from build123d import *

# Parameters (mm, degrees)
F0_W     = 50.8
F0_H     = 43.18
F1_DEPTH = 30.48
F2_R     = 16.51
F3_W     = 40.64
F3_H     = 20.32
F4_DEPTH = 38.1
F6_DEPTH = 2.54
F7_R     = 33.02
F8_R     = 9.525
F9_DEPTH = 25.4


with BuildPart() as f1:
    # F0 (on Front) → F1 (new body)
    with BuildSketch(Plane.XZ):
        with Locations((25.4, -21.59)):
            Rectangle(F0_W, F0_H)
    extrude(amount=F1_DEPTH)

    # F2
    f2_edges = [f1.edges().sort_by_distance(p)[0] for p in [
        (50.8, -15.24, -43.18),
    ]]
    fillet(f2_edges, radius=F2_R)

    # F3 (on face) → F4 (cut)
    with BuildSketch(Plane.XY):
        with Locations((25.4, -15.24)):
            Rectangle(F3_W, F3_H)
    extrude(amount=-F4_DEPTH, mode=Mode.SUBTRACT)

    # F5 (on face) → F6 (join)
    with BuildSketch(Plane(origin=(0, 0, 0), x_dir=(0, -1, 0), z_dir=(-1, 0, 0))):
        with BuildLine():
            ThreePointArc((15.24, -43.18), (21.975192, -40.390192), (24.765, -33.655))
            ThreePointArc((24.765, -33.655), (8.504808, -26.919808), (15.24, -43.18))
        make_face()
    extrude(amount=-F6_DEPTH)

    # F7
    f7_edges = [f1.edges().sort_by_distance(p)[0] for p in [
        (45.72, -15.24, -38.1),
    ]]
    fillet(f7_edges, radius=F7_R)

    # F8 (on face) → F9 (cut)
    with BuildSketch(Plane.YZ.offset(5.08)):
        with Locations((-15.24, -28.575)):
            Circle(F8_R)
    extrude(amount=-F9_DEPTH, mode=Mode.SUBTRACT)


solid = f1.part
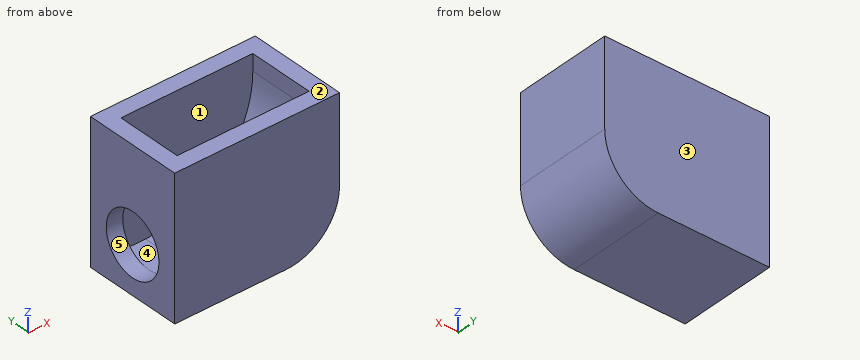
Source: CAD feature listing. Evaluate the final solid. Frame: model axes, mm. Face numbers are marked on the shaded views. A direction names the side the tool comes from. Round coordinates to 2 decimals unless told otherwise and drop trailing zeros. Loops run counter-clockwise (first coordinate to the right, second up) from the corner with the lowest first, then second, coordinate; pieces in that order, holes last. Notation, with made-up numbers: M -28,21.5 L 17,21.5 A5 ccw 17,27.5 Z; hole C 38,-13.5 d3. An arc over 180 degrees is marked long. Return JSON: item names as keys, results as strings. Group by question number.
1. Mould query, pull axis Z, two halves, no side actions, for the marked faces 3, 4 and 5. Classes: released by +Z, released by -Z, zero draft, split by the parting line, or undercut.
2. Reachability of the marked faces 1 and 2 from +Z, -Z, +X, -X, +Y, -Y: full face, straight path, thin tool, end or side. Return the list, or none.
3. Section query A-A on y = -17.5. Output: boundary loops of the cut face in (x, z), and give its area (3 significant figures).
4. Material intervals for line 1 along Z through (x, y) = (2, -15); line 2 along Y through (x, z) = (17.5, -8); line 3 along X through (y, z) = (-7, -3), sorted ascending. Write a range as from..to.
5. Section query B-B on x = 20. Output: boundary loops of the cut face in (y, z).
6. Section query C-C on z = -21. Output: boundary loops of the cut face in (x, y).
7. Pin query (flat end, axial travel): pin 1 (12 mm diameter, centred on x = 36.5, y = -13.5, fed in from +Z); pin 2 (4 mm diameter, centred on x = 8, y = -17.5, fed in from +Z). Return the tip coordinate at first contact, or that it passes through.
8. Section query D-D on y = -1.5. Output: boundary loops of the cut face in (x, z).
Checks:
{
 "1": {"face 3": "zero draft", "face 4": "released by +Z", "face 5": "undercut"},
 "2": {"face 1": "+Z", "face 2": "+Z, +X, -X, +Y, -Y"},
 "3": {"outline": "M 0,-43.18 L 34.29,-43.18 A16.51 ccw 50.8,-26.67 L 50.8,0 L 45.72,0 L 45.72,-5.08 A33.02 cw 12.7,-38.1 L 5.08,-38.1 L 5.08,-37.83 L 0,-37.83 Z; M 0,-19.32 L 5.08,-19.32 L 5.08,0 L 0,0 Z", "area": "727 mm²"},
 "4": {"line 1": "z = -43.18..-38.1, -19.05..0", "line 2": "y = -30.48..-25.4, -5.08..0", "line 3": "x = 0..5.08, 45.72..50.8"},
 "5": {"outline": "M -30.48,-43.18 L 0,-43.18 L 0,0 L -5.08,0 L -5.08,-37.28 L -25.4,-37.28 L -25.4,0 L -30.48,0 Z"},
 "6": {"outline": "M 0,-30.48 L 50.8,-30.48 L 50.8,0 L 0,0 L 0,-9.47 L 5.08,-9.47 L 5.08,-5.08 L 41.63,-5.08 L 41.63,-25.4 L 5.08,-25.4 L 5.08,-21.01 L 0,-21.01 Z"},
 "7": {"pin 1": "stops at z = -19.3", "pin 2": "stops at z = -38.1"},
 "8": {"outline": "M 0,-43.18 L 34.29,-43.18 A16.51 ccw 50.8,-26.67 L 50.8,0 L 0,0 Z"}
}
